Here's how the part is built. I have some questions about the finished solid (model axes, mm). A direction names the side the tool comes from. Round coordinates to 2 decimals unless told otherwise and drop trailing zeros. Order: outer loops, then holes, each group sorted by start corner. A loop starts at its lowest first (then second) coordinate and runs counter-clockwise, first axis right, second up. Notation, with made-up numbers: (30.5, 22.25) - (58.5, 22.25) arc R13 ccw to (58.5, 37.25) - close; hole circle Ø4 at (56, -19). An arc over 180 degrees is marked (long way). Answer as a JSON object with one key per item and string values.
```python
from build123d import *
from OCP.BRepFilletAPI import BRepFilletAPI_MakeFillet

# Parameters (mm, degrees)
BOSS_EXTRUDE1_DEPTH                                 = 15
BOSS_EXTRUDE2_DEPTH                                 = 22.5
SKETCH3_W                                           = 8
SKETCH3_H                                           = 3
BOSS_EXTRUDE3_DEPTH                                 = 3
SKETCH8_W                                           = 12
SKETCH8_H                                           = 25
CUT_EXTRUDE1_DEPTH                                  = 2
CSK_FOR_M3_COUNTERSUNK_FLAT_HEAD_SCREW1_D           = 3.4
CSK_FOR_M3_COUNTERSUNK_FLAT_HEAD_SCREW1_CSINK_D     = 6.3
CSK_FOR_M3_COUNTERSUNK_FLAT_HEAD_SCREW1_CSINK_ANGLE = 90
SKETCH9_W                                           = 12
SKETCH9_H                                           = 22.5
BOSS_EXTRUDE4_DEPTH                                 = 20
FILLET1_R                                           = 15
FILLET2_R1                                          = 1
FILLET2_R2                                          = 2
CHAMFER1_SIZE                                       = 0.6
CHAMFER2_SIZE                                       = 2


with BuildPart() as part:
    # Sketch1 → Boss-Extrude1 (new body)
    with BuildSketch(Plane(origin=(0, 0, 0), x_dir=(1, 0, 0), z_dir=(0, 1, 0))):
        Polygon((6.5, 14.5), (3, 11), (0, 11), (0, -11), (3, -11), (6.5, -14.5), (10, -11), (13, -11), (13, 11), (10, 11), align=None)
    extrude(amount=-BOSS_EXTRUDE1_DEPTH)

    # Sketch2 → Boss-Extrude2 (add)
    with BuildSketch(Plane(origin=(0, 0, 0), x_dir=(1, 0, 0), z_dir=(0, 1, 0))):
        Polygon((0, -39.25), (13, -39.25), (13, -11), (10, -11), (6.5, -14.5), (3, -11), (0, -11), align=None)
        Polygon((10, 11), (13, 11), (13, 46.25), (-81, 46.25), (-81, 36.25), (0, 36.25), (0, 11), (3, 11), (6.5, 14.5), align=None)
        Polygon((3, 11), (0, 11), (0, -11), (3, -11), (6.5, -14.5), (10, -11), (13, -11), (13, 11), (10, 11), (6.5, 14.5), align=None)
    extrude(amount=BOSS_EXTRUDE2_DEPTH)

    # Sweep1: sweep along a curve in space
    with BuildLine() as sweep1_path:
        Line((0, 22.5, 39.25), (0, 0, 39.25))
    # Sketch3 → Sweep1 (sweep)
    with BuildSketch(Plane(origin=(0, 22.5, 0), x_dir=(1, 0, 0), z_dir=(0, 1, 0))):
        with Locations((-4, -37.75)):
            Rectangle(SKETCH3_W, SKETCH3_H)
    sweep(path=sweep1_path.line)

    # Sketch4 → Boss-Extrude3 (add)
    with BuildSketch(Plane(origin=(0, 22.5, 0), x_dir=(1, 0, 0), z_dir=(0, 1, 0))):
        Polygon((-8, -36.25), (0, -36.25), (0, 36.25), (-81, 36.25), (-81, 28.25), (-8, 28.25), align=None)
    extrude(amount=-BOSS_EXTRUDE3_DEPTH)

    # Sketch8 → Cut-Extrude1 (cut)
    with BuildSketch(Plane.ZY):
        with Locations((0, 7)):
            Rectangle(SKETCH8_W, SKETCH8_H)
    extrude(amount=-CUT_EXTRUDE1_DEPTH, mode=Mode.SUBTRACT)

    # CSK for M3 Countersunk Flat Head Screw1 (through all)
    with Locations(Plane(origin=(0, 22.5, 0), x_dir=(1, 0, 0), z_dir=(0, 1, 0))):
        with Locations((6.5, 20), (6.5, -20)):
            CounterSinkHole(CSK_FOR_M3_COUNTERSUNK_FLAT_HEAD_SCREW1_D / 2, CSK_FOR_M3_COUNTERSUNK_FLAT_HEAD_SCREW1_CSINK_D / 2, counter_sink_angle=CSK_FOR_M3_COUNTERSUNK_FLAT_HEAD_SCREW1_CSINK_ANGLE)

    # Sketch9 → Boss-Extrude4 (add)
    with BuildSketch(Plane(origin=(0, 0, -46.25), x_dir=(-1, 0, 0), z_dir=(0, 0, -1))):
        with Locations((75, 11.25)):
            Rectangle(SKETCH9_W, SKETCH9_H)
    extrude(amount=BOSS_EXTRUDE4_DEPTH)

    # Fillet1
    fillet1_edges = [part.edges().sort_by_distance(p)[0] for p in [
        (-81, 9.75, -36.25),
    ]]
    fillet(fillet1_edges, radius=FILLET1_R)

    # Fillet2: one fillet with a radius per group of edges: ONE call of the kernel's fillet builder (fillet() takes one radius for all edges)
    fillet2_edges_1 = [part.edges().sort_by_distance(p)[0] for p in [
        (6.5, -7.5, -14.5),
        (6.5, -7.5, 14.5),
    ]]
    fillet2_edges_2 = [part.edges().sort_by_distance(p)[0] for p in [
        (0, 9.75, -36.25),
    ]]
    fillet2 = BRepFilletAPI_MakeFillet(part.part.solid().wrapped)
    for e in fillet2_edges_1:
        fillet2.Add(FILLET2_R1, e.wrapped)
    for e in fillet2_edges_2:
        fillet2.Add(FILLET2_R2, e.wrapped)
    add(Compound.cast(fillet2.Shape()), mode=Mode.REPLACE)

    # Chamfer1
    chamfer1_edges = [part.edges().sort_by_distance(p)[0] for p in [
        (1.5, 0, -11),
        (8.2, 0, -20),
        (8.603553391, 0, -12.396446609),
        (8.2, 0, 20),
        (11.5, 0, -11),
        (-69, 0, -56.25),
        (-75, 0, -66.25),
        (11.5, 0, 11),
        (4.396446609, -15, 12.396446609),
        (4.396446609, 0, 12.396446609),
        (-76.606601718, 0, -40.643398282),
        (1.5, 0, 11),
        (-34, 0, -36.25),
        (4.396446609, 0, -12.396446609),
        (4.396446609, -15, -12.396446609),
        (8.603553391, -15, 12.396446609),
        (6.5, -15, 14.085786438),
        (6.5, -15, -14.085786438),
        (8.603553391, 0, 12.396446609),
        (-0.585786438, 0, -35.664213562),
        (6.5, 0, -14.085786438),
        (6.5, 0, 14.085786438),
        (0, -7.5, -11),
        (13, -7.5, -11),
        (13, -7.5, 11),
        (0, -7.5, 11),
        (11.5, -15, 11),
        (13, -15, 0),
        (11.5, -15, -11),
        (2.5, 0, 39.25),
        (8.603553391, -15, -12.396446609),
        (0, 0, -22.625),
        (2.5, 22.5, 39.25),
        (13, 0, 25.125),
        (13, 0, -28.625),
        (-28, 0, -46.25),
        (-81, 0, -58.75),
        (13, 22.5, -3.5),
        (-28, 22.5, -46.25),
        (-81, 22.5, -47.25),
        (1.5, -15, -11),
        (0, -15, 0),
        (0, 0, 23.625),
        (-8, 22.5, 5.5),
        (-4, 0, 36.25),
        (-8, 0, 37.75),
        (-44.5, 22.5, -28.25),
        (1.5, -15, 11),
    ]]
    chamfer(chamfer1_edges, length=CHAMFER1_SIZE)

    # Chamfer2
    chamfer2_edges = [part.edges().sort_by_distance(p)[0] for p in [
        (2, -5.5, 0),
    ]]
    chamfer(chamfer2_edges, length=CHAMFER2_SIZE - 0.0001)  # a hair under: the kernel refuses the full size


solid = part.part
```
1. Imagine slicing it at B-B (z = -20). List the corners of the cut face in (x, y) for me.
Responses:
{"outline": "(-8, 19.5) - (0, 19.5) - (0, 0.6) - (0.6, 0) - (4.2, 0) - (4.8, 0.6) - (4.8, 21.05) - (3.35, 22.5) - (-7.4, 22.5) - (-8, 21.9) - close; (8.2, 0.6) - (8.8, 0) - (12.4, 0) - (13, 0.6) - (13, 21.9) - (12.4, 22.5) - (9.65, 22.5) - (8.2, 21.05) - close"}
2. Imagine slicing it at A-A (y = 11.5). List the corners of the cut face in (x, z) for me.
Responses:
{"outline": "(-81, -66.25) - (-69, -66.25) - (-69, -46.25) - (13, -46.25) - (13, 39.25) - (-8, 39.25) - (-8, 36.25) - (0, 36.25) - (0, 6) - (2, 6) - (2, -6) - (0, -6) - (0, -34.25) arc R2 cw to (-2, -36.25) - (-66, -36.25) arc R15 ccw to (-81, -51.25) - close; hole circle Ø3.4 at (6.5, -20); hole circle Ø3.4 at (6.5, 20)"}
3. Imagine slicing it at C-C (x = -49.5). List the corners of the cut face in (y, z) for me, plus the area to 3 significant figures.
Responses:
{"outline": "(0, -45.65) - (0.6, -46.25) - (21.9, -46.25) - (22.5, -45.65) - (22.5, -28.85) - (21.9, -28.25) - (19.5, -28.25) - (19.5, -36.25) - (0.6, -36.25) - (0, -36.85) - close", "area": "248 mm2"}
4. For P1, Ø0.6, axis at x = 1.5, y = 2.5, coming from the -Z side; P2, Ø13, axis at y = 9, z = 0, coming from the -X side; P3, Ø1.9, axis at x = 2.5, y = -5, coming from the +Z side; P4, Ø2.5, axis at x = 6.5, z = -20, coming from the +Y side, each with a flat end and sliding along its axis, tell me the tip position at first contact or that it passes through.
Responses:
{"P1": "z = -46.25", "P2": "x = 0", "P3": "z = 11.45", "P4": "through"}
5. Thinking about a two-plate mould opening in Z: for faces 1 (the face through (-0.488, 0.438, -35.796)), 2 (the face through (8.461, -14.696, 12.12)), 3 (the face through (-81, 13, -55)), which applies, pulls with the +Z half, pulls with the -Z half, needs draft (parallel to the pull), parting line crosses it, or undercut?
Responses:
{"face 1": "undercut", "face 2": "pulls with the +Z half", "face 3": "needs draft"}
6. For faces 4 (the face through (4, -7, -12)), 5 (the face through (9, -7, -12)), 6 (the face through (4, -7, 12)), which set-ups out of +Z, -Z, +X, -X, +Y, -Y let a thin tool reach every point of the face, with its end or its side?
Responses:
{"face 4": "-Z, -X, -Y", "face 5": "-Z, +X, -Y", "face 6": "+Z, -X, -Y"}
7. If I drill on L1, parallel to Z at x = 6.5, y = 7; L2, parallel to X at y = 13.75, z = 20; L3, parallel to Z at x = 6, y = 5, over which ranges is the centre line in solid material (lowest first)? Write a range as [from, to].
Responses:
{"L1": "[-46.25, -21.7], [-18.3, 18.3], [21.7, 39.25]", "L2": "[0, 4.8], [8.2, 13]", "L3": "[-46.25, -21.62], [-18.38, 18.38], [21.62, 39.25]"}
